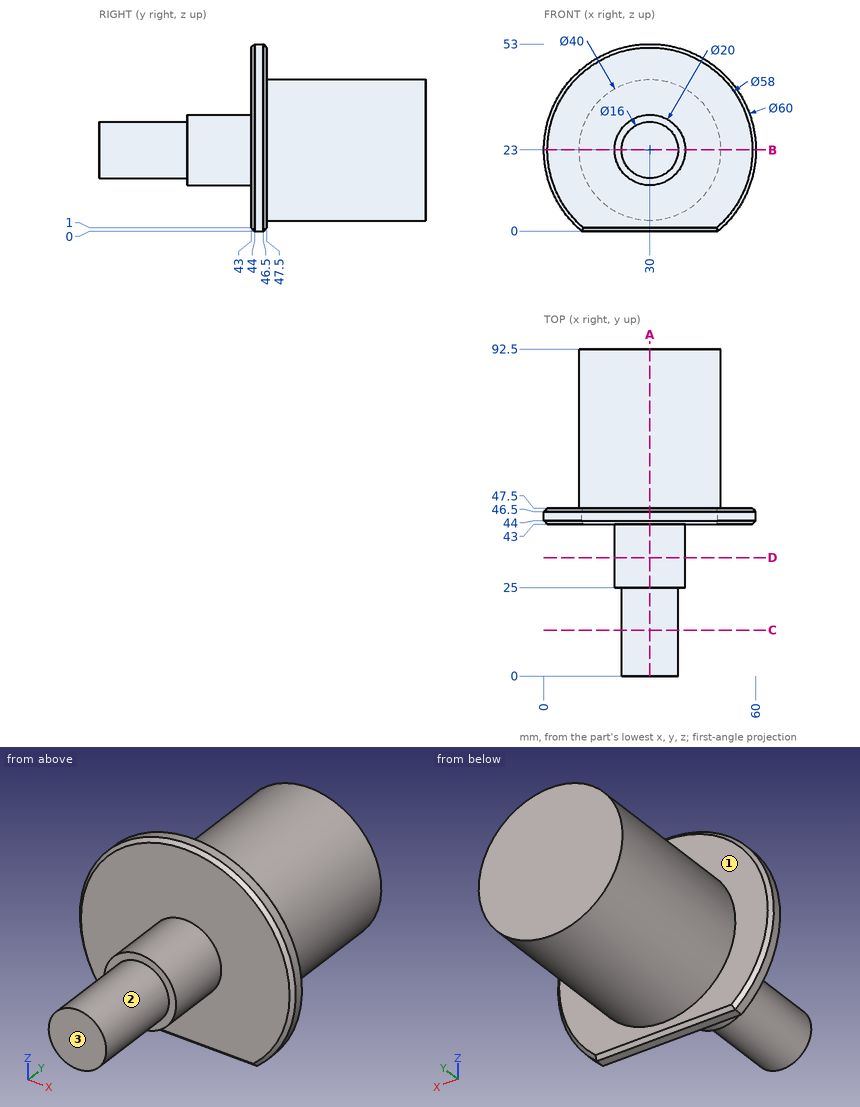
The drawing under review shows one solid part. Ordinate dimensions are in mm from its lowest x, y, z. A direction names the side the tool comes from. Round coordinates to 2 decimals unless told otherwise and drop trailing zeros. Loops run counter-clockwise (first coordinate to the right, second up) from the corner with the lowest first, then second, coordinate; pieces in that order, holes last. Notation, with made-up numbers: (35.25, 69.25) - (84.25, 69.25) arc R29 cw to (84.25, 95.25) - close; hole circle Ø9 at (-16, -38.5). An arc over 180 degrees is marked (long way). Use a Markdown table: item, result. Add a question column.
Q1. Add section A-A (x = 30). State the section outline as (y, z) points, plus the area to 3 significant figures.
Q2. Machinability: for the marked faces 1, 2 and 3, which of the approach directions +Z, -Z, +X, -X, +Y, -Y give a long, thin tool a straight path to every point of the face, cutting with its end or side? Answer none if there is none.
Q3. Add section B-B (z = 23). State the section outline as (x, y) points, plus the area to 3 significant figures.
Q4. Insertion check: pin 1 Ø2 at (x, y) = (18.5, 27.5) entering from +Z; pin 2 Ø12 at (x, y) = (20, 21) entering from +Z; pin 3 Ø2 at (y, z) = (72, 15) entering from +X (3 decimals); pin 4 Ø6 at (x, z) = (44, 16.5) entering from -Y. Each pin has a flat end and moves straight along its axis. Give the tip position at first contact, or say it passes through.
Q5. Add section D-D (y = 33.5). State the section outline as (x, z) points.
Q6. For probe 1 along X at (y, z) = (47, 28.5); probe 2 along Z at (x, y) = (29.5, 63); probe 3 along Y at (x, z) = (52, 32.5), list the stretches that pass through material, from the lowest coordinate up.
Q7. Add section C-C (y = 13). State the section outline as (x, z) points, plus the area to 3 significant figures.
Worked answers:
| question | item | result |
|---|---|---|
| 1 | outline | (0, 15) - (25, 15) - (25, 13) - (43, 13) - (43, 1) - (44, 0) - (46.5, 0) - (47.5, 1) - (47.5, 3) - (92.5, 3) - (92.5, 43) - (47.5, 43) - (47.5, 52) - (46.5, 53) - (44, 53) - (43, 52) - (43, 33) - (25, 33) - (25, 31) - (0, 31) - close |
| 1 | area | 2,800 mm² |
| 2 | face 1 | +Y |
| 2 | face 2 | -Y |
| 2 | face 3 | +Z, -Z, +X, -X, -Y |
| 3 | outline | (0, 44) - (1, 43) - (20, 43) - (20, 25) - (22, 25) - (22, 0) - (38, 0) - (38, 25) - (40, 25) - (40, 43) - (59, 43) - (60, 44) - (60, 46.5) - (59, 47.5) - (50, 47.5) - (50, 92.5) - (10, 92.5) - (10, 47.5) - (1, 47.5) - (0, 46.5) - close |
| 3 | area | 2,830 mm² |
| 4 | pin 1 | through |
| 4 | pin 2 | z = 31.33 |
| 4 | pin 3 | x = 48.735 |
| 4 | pin 4 | y = 43 |
| 5 | outline | circle Ø20 at (30, 23) |
| 6 | probe 1 | 1.02 to 58.98 |
| 6 | probe 2 | 3.01 to 42.99 |
| 6 | probe 3 | 43 to 47.5 |
| 7 | outline | circle Ø16 at (30, 23) |
| 7 | area | 201 mm² |
